Verification items for this drawing (mm, ordinates from the low corner). Round coordinates to 2 decimals unless told otherwise and drop trailing zeros. Loops run counter-clockwise (first coordinate to the right, second up) from the corner with the lowest first, then second, coordinate; pieces in that order, holes last. Notation, with made-up numbers: (68.25, 61) -> (118.25, 61) arc R26 cw to (118.25, 86) -> close; hole circle Ø7 at (42.25, -33.75). An arc over 180 degrees is marked (long way). One line per item, written item: value. Start each with the question number.
1. Cross-section at B-B on x = 102.5. Record the cut outline in (y, z), then the cut area to 3 significant figures.
2. Material ranges on L1, parallel to X at y = 118.5, z = 26; L2, parallel to X at y = 75.5, z = 9.5; L3, parallel to Y at x = 84, z = 37.5, recorded low to high.
3. Go/stop test with a flat-tipped pin: pin 1 (1 mm diameter, centred on x = 187.5, y = 141, fed in from -Z). Record where the tip stops, or that it passes through.
4. Release check for a two-part mould opening along X. For the marked faces 1, 2 and 3 record: +X half, -X half, draft (parallel to the pull), parting line (faces both ways), or undercut.
5. Cross-section at A-A on y = 83.5. Record the cut outline in (x, z), then the cut area to 3 significant figures.
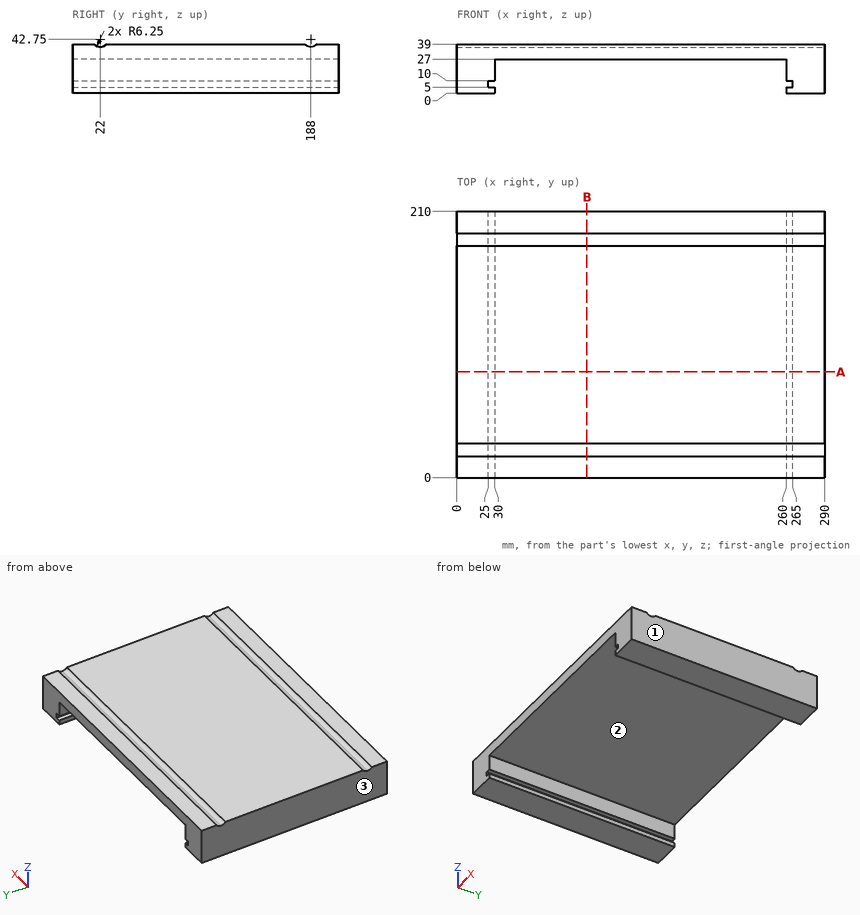
Taken from the geometry:
1. outline: (0, 27) -> (210, 27) -> (210, 39) -> (193, 39) arc R6.25 cw to (183, 39) -> (27, 39) arc R6.25 cw to (17, 39) -> (0, 39) -> close
1. area: 2,490 mm2
2. L1: x = 0 to 30, 260 to 290
2. L2: x = 0 to 25, 265 to 290
2. L3: y = 0 to 18.61, 25.39 to 184.61, 191.39 to 210
3. pin 1: stops at z = 27
4. face 1: +X half
4. face 2: undercut
4. face 3: -X half
5. outline: (0, 0) -> (30, 0) -> (30, 5) -> (25, 5) -> (25, 10) -> (30, 10) -> (30, 27) -> (260, 27) -> (260, 10) -> (265, 10) -> (265, 5) -> (260, 5) -> (260, 0) -> (290, 0) -> (290, 39) -> (0, 39) -> close
5. area: 5,050 mm2
